Source: CAD feature listing. Evaluate the final solid. Frame: model axes, mm. Give positions to 0.01 mm unless a question says otherwise; leave off trailing zeros. Return JSON: item names as keys, results as strings. Group by question number.
(1) Draft query along Y for faces 1 (the face through (-12, 92, -0.203)), 2 (the face through (-105.694, 191.665, -1.724)). Return one class per face: released by +Y, released by -Y, zero draft, split by the parting line, or undercut.
(2) Ray query, line 1 (Y direction, x = 91, z = -0.9); line 2 (X direction, y = 193.5, z = -2.9); line 3 (Y direction, x = -69, z = -1.3). Return the intervals inside material, ascending. Write a range as from..to.
(3) Pin query (flat end, axial travel): pin 1 (6.5 mm diameter, centred on x = 91, y = 6.49, fed in from +Z). Return the tip coordinate at first contact, or that it passes through.
Autodesk Inventor part; units mm, degrees
ref_plane "YZ Plane" through (0, 0, 0) normal (1, 0, 0) x (0, 1, 0)
ref_plane "XZ Plane" through (0, 0, 0) normal (0, 1, 0) x (-1, 0, 0)
ref_plane "XY Plane" through (0, 0, 0) normal (0, 0, 1) x (1, 0, 0)
ref_plane "Work Plane1" through (-9, 0, -3.2032) normal (0, 0, 1) x (1, 0, 0)
sketch "Sketch1" plane through (-9, 0, -3.2032) normal (0, 0, 1) x (1, 0, 0)
  ellipse E0 centre (-38.5, 0) end of major axis (-36.433, 0) minor radius 2.0669
  ellipse E1 centre (36.5, 0) end of major axis (38.567, 0) minor radius 2.0669
  line L0 (89, -44.9989) -> (89, 224.9989)
  line L1 (-111, 224.9989) -> (-111, -44.9989)
  line L2 (-111, -44.9989) -> (89, -44.9989)
  line L3 (89, 224.9989) -> (-91, 224.9989)
  line L4 (-91, -24.9989) -> (-91, 224.9989)
  line L5 (-91, -24.9989) -> (89, -24.9989)
  line L6 (89, 224.9989) -> (89, -24.9989)
  line L7 (-91, 224.9989) -> (-111, 224.9989)
  line L8 (89, -44.9989) -> (109, -44.9989)
  line L9 (109, -44.9989) -> (109, 224.9989)
  line L10 (109, 224.9989) -> (89, 224.9989)
  line L11 (89, 224.9989) -> (-91, 224.9989)
  point P0 (9, 0)
  point P1 (79, 224.9989)
  point P2 (79, -24.9989)
  point P3 (-81, 224.9989)
  point P4 (-81, -24.9989)
  point P5 (-91, 1846.3654)
  dimension "d40" = 20
  dimension "d41" = 90
extrude "Extrusion1" add sketch "Sketch1" along normal blind 3 contours E0 | E1 | L2 L1 L7 L4 L5 L0 | L0 L10 L9 L8 | L5 L4 L3 L0
sketch "Sketch2" plane through (-9, 0, -0.2032) normal (0, 0, 1) x (1, 0, 0)
  line L0 (-111, -44.9989) -> (89, -44.9989) construction
  line L1 (55.5, -44.9989) -> (55.5, 235.0161) construction
  line L2 (89, -44.9989) -> (89, 224.9989) construction
  line L3 (88.5, -24.9989) -> (88.5, 475.0011)
  point P0 (9, 0)
  point P1 (89, 4927.5367)
  point P2 (55.5, 105.0011)
  dimension "d4" = 33
  dimension "d12" = 150
hole "Hole1" at (46.5, 105.0011, -0.2032) direction (0, 0, -1) diameter 5.1 depth 3
sketch "Sketch3" plane through (-9, 0, -0.2032) normal (0, 0, 1) x (1, 0, 0)
  line L0 (89, -24.9989) -> (89, -24.9989)
  line L1 (89, -24.9989) -> (89, 475.0011)
  line L2 (89, 475.0011) -> (89, 475.0011)
  line L3 (89, -24.9989) -> (89, 475.0011)
  line L4 (69, -24.9989) -> (69, -24.9989)
  line L5 (69, -24.9989) -> (69, 475.0011)
  line L6 (69, 475.0011) -> (69, 475.0011)
  line L7 (69, -24.9989) -> (69, 475.0011)
  line L8 (-91, -24.9989) -> (-91, -24.9989)
  line L9 (-91, -24.9989) -> (-91, 475.0011)
  line L10 (-91, 475.0011) -> (-91, 475.0011)
  line L11 (-91, -24.9989) -> (-91, 475.0011)
  line L12 (-71, -24.9989) -> (-71, -24.9989)
  line L13 (-71, -24.9989) -> (-71, 475.0011)
  line L14 (-71, 475.0011) -> (-71, 475.0011)
  line L15 (-71, -24.9989) -> (-71, 475.0011)
  line L16 (100, -24.9989) -> (100, 239.9989) construction
  line L17 (-102, -24.9989) -> (-102, 244.9989) construction
  line L18 (-60, -24.9989) -> (-60, 2205.8354) construction
  line L19 (98.966, 4926.9545) -> (-101.034, 1503.4308) construction
  line L20 (55.3, -24.9989) -> (55.3, 4179.4968) construction
  line L21 (89, -44.9989) -> (89, 224.9989)
  point P0 (9, 0)
  point P1 (89, 4927.5367)
  point P2 (-111, 1504.013)
  point P3 (100, 6.4871)
  point P4 (-60, 126.3923)
  point P5 (-102, 57.9278)
  point P6 (-102, 193.5737)
  dimension "d14" = 11
  dimension "d15" = 11
  dimension "d16" = 13.7
  dimension "d39" = 11
hole "Hole3" at (91, 6.4871, -0.2032) at (-69, 126.3923, -0.2032) at (-111, 57.9278, -0.2032) direction (0, 0, -1) diameter 5.1 depth 3
sketch "Sketch4" plane through (-9, 0, -0.2032) normal (0, 0, 1) x (1, 0, 0)
  point P0 (9, 0)
  point P1 (-93.7009, 193.5736)
hole "Hole4" at (-102.7009, 193.5736, -0.2032) direction (0, 0, -1) diameter 7.1 depth 3
properties part number "Z axis front plate"
Answers:
{
 "1": {"face 1": "zero draft", "face 2": "undercut"},
 "2": {"line 1": "-45..3.94, 9.04..225", "line 2": "-120..-106.25, -99.15..100", "line 3": "-45..123.84, 128.94..225"},
 "3": {"pin 1": "z = -0.2"}
}
